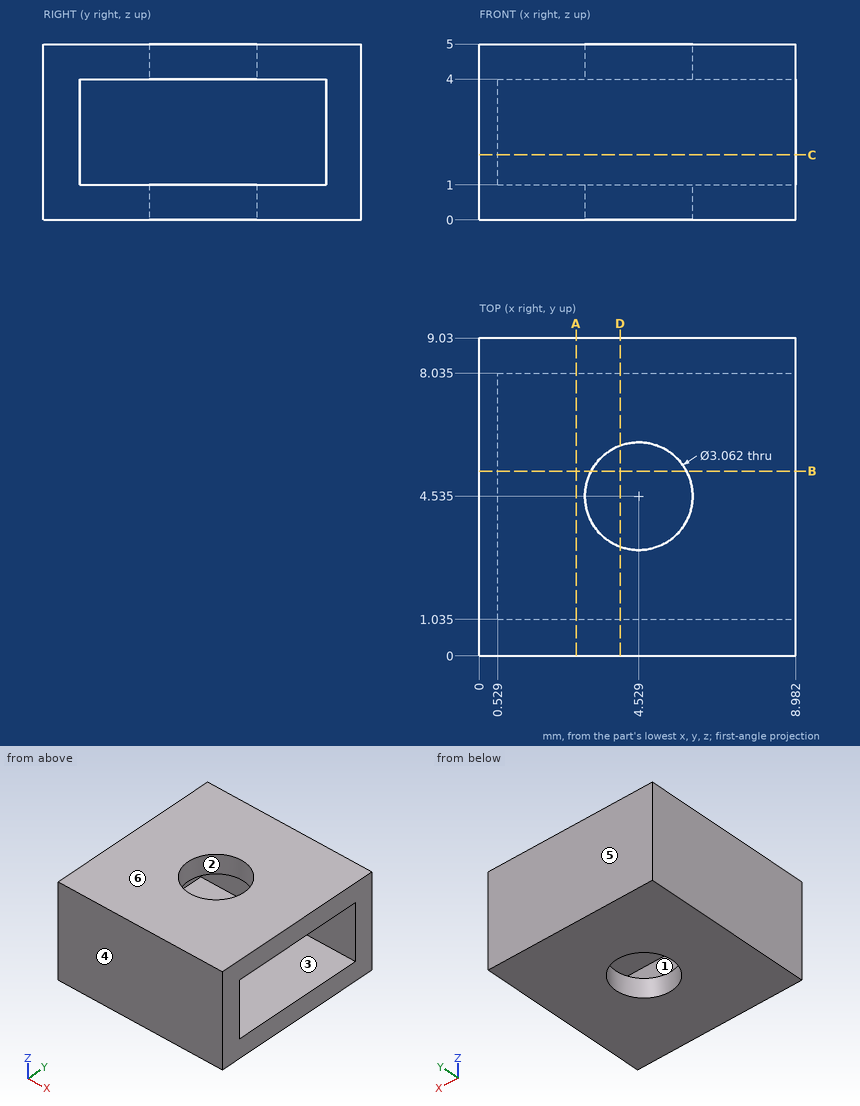
Print and shaded views of the part. All mm, measured from the part's lowest x, y and z. A direction names the side the tool comes from. Round coordinates to 2 decimals unless told otherwise and drop trailing zeros. Order: outer loops, then holes, each group sorted by start corner. A loop starts at its lowest first (then second) coordinate and runs counter-clockwise, first axis right, second up. Notation, with made-up numbers: (52, -7.75) - (108, -7.75) arc R22 cw to (108, 4.25) - close; hole circle Ø1 at (-11, 86). An arc over 180 degrees is marked (long way). Use a Markdown table: item, result.
1) Wall check: L1, parallel to Y at x = 4, z = 1.85 (1 decimal); L2, parallel to Z at x = 6, y = 8; L3, parallel to X at y = 6.5, z = 3.8. Give the ranges that are in metal, low to high.
Recorded:
| item | result |
|---|---|
| L1 | y = 0 to 1, 8 to 9 |
| L2 | z = 0 to 1, 4 to 5 |
| L3 | x = 0 to 0.53 |
2) Saw through at D-D on x = 4. Write the cut outline in (y, z) (1 decimal).
Recorded:
| item | result |
|---|---|
| outline | (0, 0) - (3.1, 0) - (3.1, 1) - (1, 1) - (1, 4) - (3.1, 4) - (3.1, 5) - (0, 5) - close; (6, 0) - (9, 0) - (9, 5) - (6, 5) - (6, 4) - (8, 4) - (8, 1) - (6, 1) - close |
3) Saw through at B-B on y = 5.25. Write the cut outline in (x, z) (1 decimal).
Recorded:
| item | result |
|---|---|
| outline | (0, 0) - (3.2, 0) - (3.2, 1) - (0.5, 1) - (0.5, 4) - (3.2, 4) - (3.2, 5) - (0, 5) - close; (5.9, 0) - (9, 0) - (9, 1) - (5.9, 1) - close; (5.9, 4) - (9, 4) - (9, 5) - (5.9, 5) - close |
4) Saw through at C-C on z = 1.85. Write the cut outline in (x, y) (1 decimal).
Recorded:
| item | result |
|---|---|
| outline | (0, 0) - (9, 0) - (9, 1) - (0.5, 1) - (0.5, 8) - (9, 8) - (9, 9) - (0, 9) - close |
5) Tool access for the marked faces 1 and 2: list every direction of +Z, -Z, +X, -X, +Y, -Y with a clear straight run to the whole face (end or side of a thin tool).
Recorded:
| item | result |
|---|---|
| face 1 | +X |
| face 2 | +Z, -Z |
6) Saw through at A-A on x = 2.75. Write the cut outline in (y, z) (1 decimal).
Recorded:
| item | result |
|---|---|
| outline | (0, 0) - (9, 0) - (9, 5) - (0, 5) - close; hole (1, 1) - (8, 1) - (8, 4) - (1, 4) - close |
7) Pull direction Y, two halves, no side cores. Call the marked faces 3, 4, 5 and 6: pulls with the +Y half, pulls with the -Y half, needs draft (parallel to the pull), parting line crosses it, or undercut.
Recorded:
| item | result |
|---|---|
| face 3 | undercut |
| face 4 | pulls with the -Y half |
| face 5 | pulls with the +Y half |
| face 6 | needs draft |
8) Flat gauge pin, fed straight in: pin 1 Ø0.9 at (y, z) = (3.5, 2) entering from +X. Where does the tip first touch, or does it go through?
Recorded:
| item | result |
|---|---|
| pin 1 | stops at x = 0.53 |
